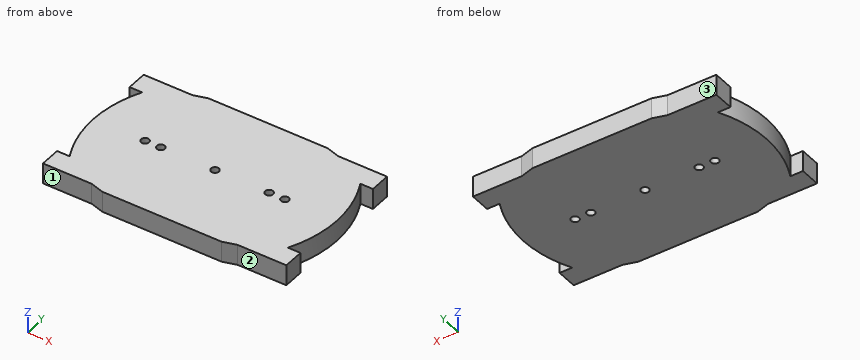
from build123d import *

# Parameters (mm, degrees)
SKETCH_1_W          = 155
SKETCH_1_H          = 98
EXTRUDE_1_DEPTH     = 13.2
CUT_EXTRUDE_1_DEPTH = 93.636331965
CUT_EXTRUDE_2_DEPTH = 93.636331965
SKETCH_4_R          = 2.5
CUT_EXTRUDE_3_DEPTH = 13.2


with BuildPart() as part:
    # 草图1 → 凸台-拉伸1 (new body)
    with BuildSketch(Plane.XY):
        Rectangle(SKETCH_1_W, SKETCH_1_H)
    extrude(amount=EXTRUDE_1_DEPTH)

    # 草图2 → 切除-拉伸1 (cut, through all)
    with BuildSketch(Plane.XY.offset(13.2)):
        Polygon((-38, 49), (-46.5, 46.5), (-77.5, 46.5), (-77.5, 49), align=None)
        Polygon((77.5, 49), (38, 49), (46.5, 46.5), (77.5, 46.5), align=None)
        Polygon((38, -49), (46.5, -46.5), (77.5, -46.5), (77.5, -49), align=None)
        Polygon((-77.5, -49), (-38, -49), (-46.5, -46.5), (-77.5, -46.5), align=None)
    extrude(amount=-CUT_EXTRUDE_1_DEPTH, mode=Mode.SUBTRACT)

    # 草图3 → 切除-拉伸2 (cut, through all)
    with BuildSketch(Plane.XY.offset(13.2)):
        with BuildLine():
            Line((-77.5, -33.5), (-69.5, -33.5))
            ThreePointArc((-69.5, -33.5), (-77.49, 0), (-69.5, 33.5))
            Line((-69.5, 33.5), (-77.5, 33.5))
            Line((-77.5, 33.5), (-77.5, -33.5))
        make_face()
        with BuildLine():
            Line((77.5, -33.5), (77.5, 33.5))
            Line((77.5, 33.5), (69.5, 33.5))
            ThreePointArc((69.5, 33.5), (77.49, 0), (69.5, -33.5))
            Line((69.5, -33.5), (77.5, -33.5))
        make_face()
    extrude(amount=-CUT_EXTRUDE_2_DEPTH, mode=Mode.SUBTRACT)

    # 草图4 → 切除-拉伸3 (cut)
    with BuildSketch(Plane(origin=(0, 0, 0), x_dir=(-1, 0, 0), z_dir=(0, 0, -1))):
        with Locations((-44.5, 0)):
            Circle(SKETCH_4_R)
        with Locations((-34.5, 0)):
            Circle(SKETCH_4_R)
        Circle(SKETCH_4_R)
        with Locations(Location((34.5, 0, 0), (0, 0, 180))):
            Circle(SKETCH_4_R)
        with Locations(Location((44.5, 0, 0), (0, 0, 180))):
            Circle(SKETCH_4_R)
    extrude(amount=-CUT_EXTRUDE_3_DEPTH, mode=Mode.SUBTRACT)


solid = part.part
The listing builds one solid part. Answer for the finished solid, in the listing's coordinates (mm). Face numbers are marked on the shaded views. A direction names the side the tool comes from. Round coordinates to 2 decimals unless told otherwise and drop trailing zeros. Write each loop counter-clockwise with the first axis right and the second up, starting at its lowest first coordinate (ties: lowest second). Pieces come first, ordered by that corner, then holes. Notation, with made-up numbers: (85, -6.75) - (131, -6.75) arc R28 ccw to (131, 32.25) - close; hole circle Ø8 at (55.5, 18.5). An arc over 180 degrees is marked (long way). Use a Markdown table: item, result. Add a question column.
1. The part is cut by section D-D (x = 68). Write down the section's boundary in (y, z).
2. The part is cut by section A-A (y = 0). Write down the section's boundary in (x, z).
3. The part is cut by section C-C (z = 7.25). Write down the section's boundary in (x, y).
4. Flat-ended cylindrical pins translate along their axes: P1, Ø1.5, axis at y = -10, z = 9.5, coming from the +X side; P2, Ø4, axis at x = -74, z = 4, coming from the +Y side; P3, Ø8, axis at x = 39, y = -10.5, coming from the -Z side; P4, Ø2.5, axis at x = 72.5, z = 4.5, coming from the -Y side. Find the tip coordinate at first contact, or state that the pin passes through.
5. Consider line 1 (Y direction, x = -34.5, z = 4.5); line 2 (Y direction, x = 44.5, z = 5.5); line 3 (X direction, y = -1.5, z = 2). Determine where each line is inside the solid, lowest interval first.
6. A tool of negligible diameter and unlimited length cuts with its end or side. For the marked faces 1, 2 and 3, from which of +Z, -Z, +X, -X, +Y, -Y can it reach the whole face along a straight path? Write none if from no direction.
7. The part is cut by section B-B (x = 0). Write down the section's boundary in (y, z), and give its area (3 significant figures).
Reported:
| question | item | result |
|---|---|---|
| 1 | outline | (-46.5, 0) - (46.5, 0) - (46.5, 13.2) - (-46.5, 13.2) - close |
| 2 | outline | (-77.49, 0) - (-47, 0) - (-47, 13.2) - (-77.49, 13.2) - close; (-42, 0) - (-37, 0) - (-37, 13.2) - (-42, 13.2) - close; (-32, 0) - (-2.5, 0) - (-2.5, 13.2) - (-32, 13.2) - close; (2.5, 0) - (32, 0) - (32, 13.2) - (2.5, 13.2) - close; (37, 0) - (42, 0) - (42, 13.2) - (37, 13.2) - close; (47, 0) - (77.49, 0) - (77.49, 13.2) - (47, 13.2) - close |
| 3 | outline | (-77.5, -46.5) - (-46.5, -46.5) - (-38, -49) - (38, -49) - (46.5, -46.5) - (77.5, -46.5) - (77.5, -33.5) - (69.5, -33.5) arc R74.22 ccw to (69.5, 33.5) - (77.5, 33.5) - (77.5, 46.5) - (46.5, 46.5) - (38, 49) - (-38, 49) - (-46.5, 46.5) - (-77.5, 46.5) - (-77.5, 33.5) - (-69.5, 33.5) arc R74.22 ccw to (-69.5, -33.5) - (-77.5, -33.5) - close; hole circle Ø5 at (-44.5, 0); hole circle Ø5 at (-34.5, 0); hole circle Ø5 at (0, 0); hole circle Ø5 at (34.5, 0); hole circle Ø5 at (44.5, 0) |
| 4 | P1 | x = 76.91 |
| 4 | P2 | y = 46.5 |
| 4 | P3 | z = 0 |
| 4 | P4 | y = -46.5 |
| 5 | line 1 | -49 to -2.5, 2.5 to 49 |
| 5 | line 2 | -47.09 to -2.5, 2.5 to 47.09 |
| 5 | line 3 | -77.47 to -46.5, -42.5 to -36.5, -32.5 to -2, 2 to 32.5, 36.5 to 42.5, 46.5 to 77.47 |
| 6 | face 1 | +Z, -Z, -X, -Y |
| 6 | face 2 | +Z, -Z, +X, -Y |
| 6 | face 3 | +Z, -Z, -X, +Y |
| 7 | outline | (-49, 0) - (-2.5, 0) - (-2.5, 13.2) - (-49, 13.2) - close; (2.5, 0) - (49, 0) - (49, 13.2) - (2.5, 13.2) - close |
| 7 | area | 1,230 mm^2 |
